Geometry check sheet. Reference: the model listing, model coordinates, mm. Give positions to 0.01 mm unless a question says otherwise; leave off trailing zeros. Loops run counter-clockwise (first coordinate to the right, second up) from the corner with the lowest first, then second, coordinate; pieces in that order, holes last. Notation, with made-up numbers: (29.25, 32) - (57.25, 32) arc R17 cw to (57.25, 54) - close; hole circle Ø9 at (-11.5, 29). An arc over 180 degrees is marked (long way). Write item = value, one per line. Start each with the question number.
from build123d import *

# Parameters (mm, degrees)
SKETCH1_W           = 250
SKETCH1_H           = 30
SKETCH1_R           = 1.75
SKETCH1_R_2         = 2
SKETCH1_R_3         = 3.25
BOSS_EXTRUDE1_DEPTH = 2


with BuildPart() as part:
    # Sketch1 → Boss-Extrude1 (new body)
    with BuildSketch(Plane(origin=(0, 0, 0), x_dir=(1, 0, 0), z_dir=(0, 1, 0))):
        Rectangle(SKETCH1_W, SKETCH1_H)
        with Locations(Location((-115, 5, 0), (0, 0, 270))):
            Circle(SKETCH1_R, mode=Mode.SUBTRACT)
        with Locations(Location((-115, -5, 0), (0, 0, 270))):
            Circle(SKETCH1_R, mode=Mode.SUBTRACT)
        with Locations(Location((0, 0, 0), (0, 0, 270))):
            Circle(SKETCH1_R, mode=Mode.SUBTRACT)
        with Locations(Location((115, 5, 0), (0, 0, 270))):
            Circle(SKETCH1_R, mode=Mode.SUBTRACT)
        with Locations(Location((115, -5, 0), (0, 0, 270))):
            Circle(SKETCH1_R, mode=Mode.SUBTRACT)
        with Locations(Location((-100.625, 0, 0), (0, 0, 270))):
            Circle(SKETCH1_R_2, mode=Mode.SUBTRACT)
        with Locations(Location((-71.875, 0, 0), (0, 0, 270))):
            Circle(SKETCH1_R_2, mode=Mode.SUBTRACT)
        with Locations(Location((-57.5, 0, 0), (0, 0, 270))):
            Circle(SKETCH1_R_2, mode=Mode.SUBTRACT)
        with Locations(Location((14.375, 0, 0), (0, 0, 270))):
            Circle(SKETCH1_R_3, mode=Mode.SUBTRACT)
        with Locations(Location((43.125, 0, 0), (0, 0, 270))):
            Circle(SKETCH1_R_3, mode=Mode.SUBTRACT)
        with Locations(Location((57.5, 0, 0), (0, 0, 270))):
            Circle(SKETCH1_R_3, mode=Mode.SUBTRACT)
        with Locations(Location((71.875, 0, 0), (0, 0, 270))):
            Circle(SKETCH1_R_3, mode=Mode.SUBTRACT)
        with Locations(Location((86.25, 0, 0), (0, 0, 270))):
            Circle(SKETCH1_R_3, mode=Mode.SUBTRACT)
        with Locations(Location((100.625, 0, 0), (0, 0, 270))):
            Circle(SKETCH1_R_3, mode=Mode.SUBTRACT)
        with Locations(Location((-43.125, 0, 0), (0, 0, 270))):
            Circle(SKETCH1_R_3, mode=Mode.SUBTRACT)
        with Locations(Location((-86.25, 0, 0), (0, 0, 270))):
            Circle(SKETCH1_R_2, mode=Mode.SUBTRACT)
        with Locations(Location((-28.75, 0, 0), (0, 0, 270))):
            Circle(SKETCH1_R_3, mode=Mode.SUBTRACT)
        with Locations(Location((-14.375, 0, 0), (0, 0, 270))):
            Circle(SKETCH1_R_3, mode=Mode.SUBTRACT)
        with Locations(Location((28.75, 0, 0), (0, 0, 270))):
            Circle(SKETCH1_R_3, mode=Mode.SUBTRACT)
    extrude(amount=BOSS_EXTRUDE1_DEPTH)


solid = part.part
1) Cross-section at B-B on y = 0.8. Give the number of separate pieces and of enclosed holes in the cut face, and give its area (3 significant figures).
2) Release check for a two-part mould opening along Z. For faces 1 (the face through (-84.267, 0.986, -0.26)), 2 (the face through (-2, 2, 0)) record: pulls with the +Z half, pulls with the -Z half, needs draft (parallel to the pull), parting line crosses it, or undercut.
3) Material ranges on line 1 along X through (y, z) = (0.7, -5.25); line 2 along Z through (x, y) = (-115, 1.2); line 3 along Z through (x, y) = (-87.5, 1.2), recorded low to high.
4) Cross-section at A-A on x = 57.5. Enter the section's corners in (y, z), and give its area (3 significant figures).
Checked values:
q1.separate_pieces = 1
q1.enclosed_holes = 19
q1.area = 7,070 mm²
q2.face_1 = undercut
q2.face_2 = needs draft
q3.line_1 = -125 to -116.73, -113.27 to 113.27, 116.73 to 125
q3.line_2 = -15 to -6.75, -3.25 to 3.25, 6.75 to 15
q3.line_3 = -15 to -1.56, 1.56 to 15
q4.outline = (0, -15) - (2, -15) - (2, -3.25) - (0, -3.25) - close; (0, 3.25) - (2, 3.25) - (2, 15) - (0, 15) - close
q4.area = 47.0 mm²
